Build history of the part. All positions in model axes, mm. A direction names the side the tool comes from. Round coordinates to 2 decimals unless told otherwise and drop trailing zeros. Order: outer loops, then holes, each group sorted by start corner. A loop starts at its lowest first (then second) coordinate and runs counter-clockwise, first axis right, second up. Notation, with made-up numbers: M -26.5,47 L -3.5,47 A13 cw -3.5,72 Z; hole C -7,27.25 d5. An arc over 180 degrees is marked long. One line per item, written item: value. Start each with the question number.
Item 1: Band-saw the part on C-C, the plane x = 0.75. Write the cut outline in (y, z), then the cut area to 3 significant figures.
Item 2: Band-saw the part on D-D, the plane z = 2.05. Write the cut outline in (x, y), then the cut area to 3 significant figures.
Item 3: Band-saw the part on B-B, the plane z = 0.5. Write the cut outline in (x, y), then the cut area to 3 significant figures.
Item 4: Two-plate mould, pull along X, no slides. Class faces 1 (the cylindrical face through (-2.58, -2.85, 1.52)), 2 (the flat face through (0, 3.452, 1)), 3 (the cylindrical face through (2.58, 2.85, 1.48)), 4 (the flat face through (1.95, 0, 1)): +X half, -X half, draft (parallel to the pull), parting line (faces both ways), or undercut.
Item 5: Tool access for faces 5 (the flat face through (-3.15, 0, 1)), 6 (the flat face through (-1, 1, 0.6)): list every direction of +Z, -Z, +X, -X, +Y, -Y with a clear straight run to the whole face (end or side of a thin tool).
Item 6: Probe L1, parallel to X at y = 1, z = 1.8; L2, parallel to Z at x = -0.75, y = 1.75; L3, parallel to Y at x = 0, z = 2.7. List the from-to ranges inside material, lowest first.
Item 7: Band-saw the part on A-A, the plane y = 0. Write the cut outline in (x, z).
```python
from build123d import *

# Parameters (mm, degrees)
F0_W     = 6.3
F0_H     = 6.903332
F0_R     = 1
F1_DEPTH = 0.6
F2_W     = 6.3
F2_H     = 6.903332
F3_DEPTH = 1.8
F4_W     = 6.3
F4_H     = 6.903332
F4_R     = 1
F5_DEPTH = 0.6
F6_R     = 2


with BuildPart() as f1:
    # F0 (on Top) → F1 (new body)
    with BuildSketch(Plane.XY):
        Rectangle(F0_W, F0_H)
        Circle(F0_R, mode=Mode.SUBTRACT)
    extrude(amount=F1_DEPTH)

    # F2 (on face) → F3 (join)
    with BuildSketch(Plane.XY.offset(0.6)):
        Rectangle(F2_W, F2_H)
        Polygon((-1.95, 1.125833), (0, 2.251666), (1.95, 1.125833), (1.95, -1.125833), (0, -2.251666), (-1.95, -1.125833), align=None, mode=Mode.SUBTRACT)
    extrude(amount=F3_DEPTH)

    # F4 (on face) → F5 (join)
    with BuildSketch(Plane.XY.offset(2.4)):
        Rectangle(F4_W, F4_H)
        Circle(F4_R, mode=Mode.SUBTRACT)
    extrude(amount=F5_DEPTH)

    # F6
    f6_edges = [f1.edges().sort_by_distance(p)[0] for p in [
        (3.15, -3.451666, 1.5),
        (3.15, 3.451666, 1.5),
        (-3.15, 3.451666, 1.5),
        (-3.15, -3.451666, 1.5),
    ]]
    fillet(f6_edges, radius=F6_R)


solid = f1.part
```
Output:
1. outline: M -3.45,0 L -0.66,0 L -0.66,0.6 L -1.82,0.6 L -1.82,2.4 L -0.66,2.4 L -0.66,3 L -3.45,3 Z; M 0.66,0 L 3.45,0 L 3.45,3 L 0.66,3 L 0.66,2.4 L 1.82,2.4 L 1.82,0.6 L 0.66,0.6 Z
1. area: 12.6 mm²
2. outline: M -3.15,-1.45 A2 ccw -1.15,-3.45 L 1.15,-3.45 A2 ccw 3.15,-1.45 L 3.15,1.45 A2 ccw 1.15,3.45 L -1.15,3.45 A2 ccw -3.15,1.45 Z; hole M -1.95,-1.13 L 0,-2.25 L 1.95,-1.13 L 1.95,1.13 L 0,2.25 L -1.95,1.13 Z
2. area: 26.9 mm²
3. outline: M -3.15,-1.45 A2 ccw -1.15,-3.45 L 1.15,-3.45 A2 ccw 3.15,-1.45 L 3.15,1.45 A2 ccw 1.15,3.45 L -1.15,3.45 A2 ccw -3.15,1.45 Z; hole C 0,0 d2
3. area: 36.9 mm²
4. face 1: -X half
4. face 2: draft
4. face 3: +X half
4. face 4: undercut
5. face 5: +Z, -Z, -X, +Y, -Y
5. face 6: none
6. L1: x = -3.15 to -1.95, 1.95 to 3.15
6. L2: z = 0 to 0.6, 2.4 to 3
6. L3: y = -3.45 to -1, 1 to 3.45
7. outline: M -3.15,0 L -1,0 L -1,0.6 L -1.95,0.6 L -1.95,2.4 L -1,2.4 L -1,3 L -3.15,3 Z; M 1,0 L 3.15,0 L 3.15,3 L 1,3 L 1,2.4 L 1.95,2.4 L 1.95,0.6 L 1,0.6 Z
